Read the model definition and answer for the solid it produces. Units are mm, in the model's axes. Round coordinates to 2 decimals unless told otherwise and drop trailing zeros. Order: outer loops, then holes, each group sorted by start corner. A loop starts at its lowest first (then second) coordinate and runs counter-clockwise, first axis right, second up. Notation, with made-up numbers: (-15.75, -19.5) - (4.25, -19.5) arc R27 ccw to (4.25, 15.5) - close; hole circle Ø11 at (-12, 73). An arc over 180 degrees is marked (long way). Put each result on its own line as item: value. Start each with the question number.
Q1. Section A-A on y = -11.5 is taken. Give the vertices of the cut face in (x, z), then the cut area to 4 significant figures.
Q2. Each of these flat-tipped pins is pushed along its axis until it touches: pin 1 Ø3 at (x, z) = (-21, 96) entering from -Y; pin 2 Ø8 at (y, z) = (-26.5, -74.5) entering from +X; pin 3 Ø8 at (y, z) = (-31, -61) entering from +X. Where does it stop, or does it pass through?
Q3. Find the intervals of material crossed by line 1 along Y through (x, z) = (-23, 90.5); line 2 along X through (y, z) = (-42.5, -27.5); line 3 along X through (y, z) = (-11, 105), in increasing order. Write a range as from..to.
from build123d import *

# Parameters (mm, degrees)
F1_DEPTH = 45
F2_R     = 5


with BuildPart() as f1:
    # F0 (on Front) → F1 (new body)
    with BuildSketch(Plane.XZ):
        Polygon((0, 175), (-85, 175), (-135, -175), (-90, -175), align=None)
    extrude(amount=F1_DEPTH)

    # F2
    f2_edges = [f1.edges().sort_by_distance(p)[0] for p in [
        (-42.5, -45, 175),
        (-110, -45, 0),
        (-112.5, -45, -175),
        (-45, -45, 0),
        (-42.5, 0, 175),
        (-110, 0, 0),
        (-112.5, 0, -175),
        (-45, 0, 0),
    ]]
    fillet(f2_edges, radius=F2_R)


solid = f1.part
Findings:
1. outline: (-135, -175) - (-90, -175) - (0, 175) - (-85, 175) - close
1. area: 22,750 mm2
2. pin 1: y = -44.12
2. pin 2: x = -63.13
2. pin 3: x = -59.66
3. line 1: -43.29..-1.71
3. line 2: -113.25..-52.76
3. line 3: -95..-18
